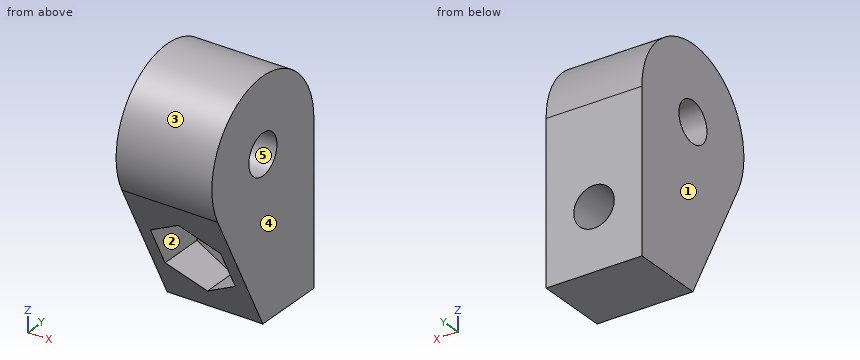
from build123d import *

# Parameters (mm, degrees)
SKETCH1_R           = 6
SKETCH1_R_2         = 1.65
BOSS_EXTRUDE1_DEPTH = 3.9
BOSS_EXTRUDE2_DEPTH = 3.9
SKETCH2_R           = 1.65
CUT_EXTRUDE5_DEPTH  = 19.116567004
CUT_EXTRUDE6_START  = 4
CUT_EXTRUDE6_DEPTH  = 15.116567004


with BuildPart() as part:
    # Sketch1 → Boss-Extrude1 (new, symmetric)
    with BuildSketch(Plane(origin=(0, 0, 0), x_dir=(0, 0, -1), z_dir=(1, 0, 0))):
        Circle(SKETCH1_R)
        Circle(SKETCH1_R_2, mode=Mode.SUBTRACT)
    extrude(amount=BOSS_EXTRUDE1_DEPTH, both=True)

    # Sketch1_4 → Boss-Extrude2 (add, symmetric)
    with BuildSketch(Plane(origin=(0, 0, 0), x_dir=(0, 0, -1), z_dir=(1, 0, 0))):
        with BuildLine():
            ThreePointArc((0, 6), (5.828221306, 1.425424992), (2.769230769, -5.322721198))
            Line((2.769230769, -5.322721198), (13, 0))
            Line((13, 0), (13, 6))
            Line((13, 6), (0, 6))
        make_face()
    extrude(amount=BOSS_EXTRUDE2_DEPTH, both=True)

    # Sketch2 → Cut-Extrude5 (cut, through all)
    with BuildSketch(Plane(origin=(0, 6, 0), x_dir=(1, 0, 0), z_dir=(0, 1, 0))):
        with Locations(Location((0, 8, 0), (0, 0, 270))):
            Circle(SKETCH2_R)
    extrude(amount=-CUT_EXTRUDE5_DEPTH, mode=Mode.SUBTRACT)

    # Sketch3 → Cut-Extrude6 (cut, through all)
    with BuildSketch(Plane.XZ.offset(-6).offset(CUT_EXTRUDE6_START)):
        Polygon((0, -11.3), (2.857883832, -9.65), (2.857883832, -6.35), (0, -4.7), (-2.857883832, -6.35), (-2.857883832, -9.65), align=None)
    extrude(amount=CUT_EXTRUDE6_DEPTH, mode=Mode.SUBTRACT)


solid = part.part
Geometry check sheet. Reference: the model listing, model coordinates, mm. Face numbers are marked on the shaded views. A direction names the side the tool comes from. Round coordinates to 2 decimals unless told otherwise and drop trailing zeros. Loops run counter-clockwise (first coordinate to the right, second up) from the corner with the lowest first, then second, coordinate; pieces in that order, holes last. Notation, with made-up numbers: (11.5, 43) -> (54.5, 43) arc R23 cw to (54.5, 73) -> close; hole circle Ø6 at (33, 83). An arc over 180 degrees is marked (long way). Answer as a JSON object with one key per item and string values. Group by question number.
Item 1: Cross-section at A-A, the plane y = -0.5. Record the cut outline in (x, z), plus the area to 3 significant figures.
Item 2: Depth check by flat-ended pin: pin 1 Ø2 at (x, z) = (1.5, -7.5) entering from -Y. Enter the tip coordinate at first touch or a pass-through.
Item 3: Release check for a two-part mould opening along Z. For the marked faces 3, 4 and 5 record: pulls with the +Z half, pulls with the -Z half, needs draft (parallel to the pull), parting line crosses it, or undercut.
Item 4: Thickness scan on line 1 along X through (y, z) = (3.4, -8); line 2 along Z through (x, y) = (-1.75, -0.75); line 3 along Y through (x, z) = (-2.5, -7). Record the ranges inside material, lowest first.
Item 5: Cross-section at C-C, the plane z = -6.75. Record the cut outline in (x, y), plus the area to 3 significant figures.
Item 6: Cross-section at D-D, the plane x = 3.25. Record the cut outline in (y, z), plus the area to 3 significant figures.
Item 7: Cross-section at B-B, the plane x = -1. Record the cut outline in (y, z).
Item 8: Set-up check for the marked faces 1 and 2: record each of +Z, -Z, +X, -X, +Y, -Y from which the full face is reachable in a straight line by a thin tool's end or side.
Determined:
{
 "1": {"outline": "(-3.9, -12.04) -> (3.9, -12.04) -> (3.9, -1.57) -> (-3.9, -1.57) -> close; (-3.9, 1.57) -> (3.9, 1.57) -> (3.9, 5.98) -> (-3.9, 5.98) -> close; hole (-2.86, -9.65) -> (0, -11.3) -> (2.86, -9.65) -> (2.86, -6.35) -> (0, -4.7) -> (-2.86, -6.35) -> close", "area": "87.7 mm²"},
 "2": {"pin 1": "stops at y = 2"},
 "3": {"face 3": "parting line crosses it", "face 4": "needs draft", "face 5": "undercut"},
 "4": {"line 1": "x = -3.9 to -1.65, 1.65 to 3.9", "line 2": "z = -11.56 to -10.29, -5.71 to -1.47, 1.47 to 5.95", "line 3": "y = 2 to 6"},
 "5": {"outline": "(-3.9, -3.25) -> (-2.86, -3.25) -> (-2.86, 2) -> (-1.08, 2) -> (-1.08, 6) -> (-3.9, 6) -> close; (1.08, 2) -> (2.86, 2) -> (2.86, -3.25) -> (3.9, -3.25) -> (3.9, 6) -> (1.08, 6) -> close", "area": "33.5 mm²"},
 "6": {"outline": "(-5.32, -2.77) -> (0, -13) -> (6, -13) -> (6, 0) arc R6 ccw (long way) to start; hole circle Ø3.3 at (0, 0)", "area": "169 mm²"},
 "7": {"outline": "(-5.32, -2.77) -> (-4.02, -5.28) -> (2, -5.28) -> (2, -6.69) -> (6, -6.69) -> (6, 0) arc R6 ccw (long way) to start; (-1.18, -10.72) -> (0, -13) -> (6, -13) -> (6, -9.31) -> (2, -9.31) -> (2, -10.72) -> close; hole circle Ø3.3 at (0, 0)"},
 "8": {"face 1": "+Z, -Z, -X, +Y, -Y", "face 2": "-Y"}
}
